Model file for the job. Use its own axes, mm. A direction names the side the tool comes from. Give positions to 0.01 mm unless a question says otherwise; leave off trailing zeros. Order: outer loops, then holes, each group sorted by start corner. A loop starts at its lowest first (then second) coordinate and runs counter-clockwise, first axis right, second up. Notation, with made-up numbers: (18, 69) - (75, 69) arc R18 cw to (75, 92) - close; hole circle Ø8 at (20, 74). An arc over 180 degrees is marked (long way). Use CSV: the item, a comma, the result in double quotes. Start each with the question number.
(1) Pull direction Z, two halves, no side cores. Call faces 1 (the flat face through (0, 0, 0)), 2 (the flat face through (0, 6, -18.745)), 3 (the cylindrical face through (-0.358, 0.986, -10.144)), 4 (the cylindrical face through (-0.22, 0.99, 10.05)): +Z half, -Z half, draft (parallel to the pull), parting line (faces both ways), or undercut.
(2) Band-saw the part on C-C, the plane z = -2.5. Give the cut face in (x, y) (3 decimals), then the cut area to 3 significant figures.
(3) Band-saw the part on B-B, the plane y = 6.5. Give the cut face in (x, z) (3 decimals).
(4) Drop flat-ended pins along their axis: pin 1 Ø2.5 at (x, z) = (0, 11.745) entering from -Y; pin 2 Ø8 at (x, z) = (14, 5) entering from -Y. Give the stop position or say it passes through.
(5) Probe L1, parallel to Z at x = 0, y = 0.85 (3 decimals); L2, parallel to Z at x = 1, y = 8.25 (3 decimals); L3, parallel to X at y = 4.5, z = 15 (3 decimals). List the from-to ranges inside material, lowest first.
(6) Band-saw the part on A-A, the plane x = 0. Give the cut face in (y, z) (3 decimals).
(7) Band-saw the part on D-D, the plane x = 12. Give the cut face in (y, z) (3 decimals).
(8) Tool access for faces 5 (the flat face through (0, 6, 18.745)), 6 (the flat face through (0, 8, 16.745)): list every direction of +Z, -Z, +X, -X, +Y, -Y with a clear straight run to the whole face (end or side of a thin tool).
from build123d import *

# Parameters (mm, degrees)
SKETCH1_W           = 52.63
SKETCH1_H           = 37.49
SKETCH1_R           = 1.65
SKETCH1_R_2         = 1.707739437
BOSS_EXTRUDE1_DEPTH = 13
SKETCH3_W           = 48.63
SKETCH3_H           = 33.49
CUT_EXTRUDE2_DEPTH  = 11


with BuildPart() as part:
    # Sketch1 → Boss-Extrude1 (new body)
    with BuildSketch(Plane(origin=(0, 0, 0), x_dir=(1, 0, 0), z_dir=(0, 1, 0))):
        Rectangle(SKETCH1_W, SKETCH1_H)
        with Locations((0, 11.755)):
            Circle(SKETCH1_R, mode=Mode.SUBTRACT)
        with Locations((0, -11.745)):
            Circle(SKETCH1_R_2, mode=Mode.SUBTRACT)
    extrude(amount=BOSS_EXTRUDE1_DEPTH)

    # Sketch3 → Cut-Extrude2 (cut)
    with BuildSketch(Plane(origin=(0, 13, 0), x_dir=(1, 0, 0), z_dir=(0, 1, 0))):
        Rectangle(SKETCH3_W, SKETCH3_H)
    extrude(amount=-CUT_EXTRUDE2_DEPTH, mode=Mode.SUBTRACT)


solid = part.part
Answer block:
1,face 1,"draft"
1,face 2,"-Z half"
1,face 3,"undercut"
1,face 4,"undercut"
2,outline,"(-26.315, 0) - (26.315, 0) - (26.315, 13) - (24.315, 13) - (24.315, 2) - (-24.315, 2) - (-24.315, 13) - (-26.315, 13) - close"
2,area,"149 mm2"
3,outline,"(-26.315, -18.745) - (26.315, -18.745) - (26.315, 18.745) - (-26.315, 18.745) - close; hole (-24.315, -16.745) - (24.315, -16.745) - (24.315, 16.745) - (-24.315, 16.745) - close"
4,pin 1,"passes through"
4,pin 2,"stops at y = 0"
5,L1,"z = -18.745 to -13.405, -10.105 to 10.037, 13.453 to 18.745"
5,L2,"z = -18.745 to -16.745, 16.745 to 18.745"
5,L3,"x = -26.315 to -24.315, 24.315 to 26.315"
6,outline,"(0, -18.745) - (13, -18.745) - (13, -16.745) - (2, -16.745) - (2, -13.405) - (0, -13.405) - close; (0, -10.105) - (2, -10.105) - (2, 10.037) - (0, 10.037) - close; (0, 13.453) - (2, 13.453) - (2, 16.745) - (13, 16.745) - (13, 18.745) - (0, 18.745) - close"
7,outline,"(0, -18.745) - (13, -18.745) - (13, -16.745) - (2, -16.745) - (2, 16.745) - (13, 16.745) - (13, 18.745) - (0, 18.745) - close"
8,face 5,"+Z, +X, -X, +Y, -Y"
8,face 6,"+Y"
